The model under review builds one solid part; all positions refer to its coordinate system, in mm. A direction names the side the tool comes from. Give positions to 0.01 mm unless a question says otherwise; leave off trailing zeros. Write each loop counter-clockwise with the first axis right and the second up, starting at its lowest first coordinate (ties: lowest second). Pieces come first, ordered by that corner, then holes. Notation, with made-up numbers: (-21.5, 70.5) -> (-7.5, 70.5) arc R13 cw to (-7.5, 80.5) -> close; hole circle Ø11 at (-7.75, 54.25). An arc over 180 degrees is marked (long way). Use CSV: the item, a comma, the result in double quotes.
Autodesk Inventor part; units mm, degrees
ref_plane "YZ Plane" through (0, 0, 0) normal (1, 0, 0) x (0, 1, 0)
ref_plane "XZ Plane" through (0, 0, 0) normal (0, 1, 0) x (-1, 0, 0)
ref_plane "XY Plane" through (0, 0, 0) normal (0, 0, 1) x (1, 0, 0)
ref_plane "Work Plane1" through (0, 0, 0) normal (0, 0, 1) x (1, 0, 0)
sketch "Sketch1" plane through (0, 0, 0) normal (0, 0, 1) x (1, 0, 0)
  arc A0 (-10.7354, 13.2764) -> (-8.7899, 5.3181) centre (6.5146, 13.2764) ccw
  line L0 (2.2646, -15.9406) -> (-8.7899, 5.3181)
  line L1 (2.2646, -15.9406) -> (17.0046, -15.9406)
  line L2 (17.0046, -15.9406) -> (17.0046, -1.0343)
  arc A1 (-5.2391, 19.424) -> (17.0046, -1.0343) centre (26.9358, 32.085) ccw
  arc A2 (-5.2391, 19.424) -> (-10.7354, 23.5341) centre (-10.7011, 17.8498) ccw
  line L3 (-10.7354, 23.5341) -> (-10.7354, 13.2764)
  line L4 (17.0046, -15.9406) -> (26.0046, -15.9406)
  line L5 (26.0046, -15.9406) -> (26.0046, 2.0594)
  line L6 (26.0046, 2.0594) -> (17.0046, 2.0594)
  line L7 (17.0046, 2.0594) -> (17.0046, -15.9406)
  line L8 (17.0046, -15.9406) -> (8.0046, -15.9406)
  line L9 (8.0046, -15.9406) -> (8.0046, 2.0594)
  line L10 (8.0046, 2.0594) -> (17.0046, 2.0594)
  line L11 (17.0046, 2.0594) -> (17.0046, -15.9406)
  point P0 (0, 0)
  dimension "d0" = 9
  dimension "d1" = 18
  dimension "d2" = 9
extrude "Extrusion1" add sketch "Sketch1" along normal blind 6 contours L9 L10 A1 L2 L1 | L10 L7 A1 | L2 L7 L6 L5 L4
sketch "Sketch2" plane through (0, 0, 6) normal (0, 0, 1) x (1, 0, 0)
  line L0 (26.0046, 2.0594) -> (8.0046, 2.0594)
  line L1 (8.0046, 2.0594) -> (8.0046, -15.9406)
  line L2 (8.0046, -15.9406) -> (26.0046, -15.9406)
  line L3 (26.0046, -15.9406) -> (26.0046, 2.0594)
  line L4 (17.0046, -15.9406) -> (17.0046, -12.4406) construction
  line L5 (17.0046, -12.4406) -> (17.0046, -2.4406) construction
  point P0 (0, 0)
  dimension "d5" = 3.5
  dimension "d6" = 10
hole "Hole1" at (17.0046, -12.4406, 6) at (17.0046, -2.4406, 6) direction (0, 0, -1) diameter 3 end through all
sketch "Sketch3" plane through (0, 0, 0) normal (0, 0, -1) x (-1, 0, 0)
  circle A0 centre (-17.0046, -12.4406) radius 1.5
  circle A1 centre (-17.0046, -2.4406) radius 1.5
  line L0 (-8.0046, -15.9406) -> (-26.0046, -15.9406)
  line L1 (-8.0046, 2.0594) -> (-8.0046, -15.9406)
  line L2 (-26.0046, 2.0594) -> (-8.0046, 2.0594)
  line L3 (-26.0046, -15.9406) -> (-26.0046, 2.0594)
  line L4 (-20.2955, -12.4406) -> (-18.65, -9.5906)
  line L5 (-18.65, -9.5906) -> (-15.3591, -9.5906)
  line L6 (-15.3591, -9.5906) -> (-13.7137, -12.4406)
  line L7 (-13.7137, -12.4406) -> (-15.3591, -15.2906)
  line L8 (-15.3591, -15.2906) -> (-18.65, -15.2906)
  line L9 (-18.65, -15.2906) -> (-20.2955, -12.4406)
  line L10 (-20.2955, -2.4406) -> (-18.65, 0.4094)
  line L11 (-18.65, 0.4094) -> (-15.3591, 0.4094)
  line L12 (-15.3591, 0.4094) -> (-13.7137, -2.4406)
  line L13 (-13.7137, -2.4406) -> (-15.3591, -5.2906)
  line L14 (-15.3591, -5.2906) -> (-18.65, -5.2906)
  line L15 (-18.65, -5.2906) -> (-20.2955, -2.4406)
  point P0 (0, 0)
  dimension "d14" = 5.7
ref_plane "Work Plane2" through (0, 0, 3.5) normal (0, 0, -1) x (-1, 0, 0)
sketch "Sketch4" plane through (0, 0, 3.5) normal (0, 0, -1) x (-1, 0, 0)
  line L0 (-18.65, 0.4094) -> (-15.3591, 0.4094)
  line L1 (-20.2955, -2.4406) -> (-18.65, 0.4094)
  circle A0 centre (-17.0046, -2.4406) radius 1.5
  circle A1 centre (-17.0046, -12.4406) radius 1.5
  line L2 (-15.3591, -5.2906) -> (-18.65, -5.2906)
  line L3 (-18.65, -9.5906) -> (-15.3591, -9.5906)
  line L4 (-20.2955, -12.4406) -> (-18.65, -9.5906)
  line L5 (-20.2955, -12.4406) -> (-18.65, -9.5906)
  line L6 (-18.65, -9.5906) -> (-15.3591, -9.5906)
  line L7 (-15.3591, -9.5906) -> (-13.7137, -12.4406)
  line L8 (-13.7137, -12.4406) -> (-15.3591, -15.2906)
  line L9 (-15.3591, -15.2906) -> (-18.65, -15.2906)
  line L10 (-18.65, -15.2906) -> (-20.2955, -12.4406)
  line L11 (-20.2955, -2.4406) -> (-18.65, 0.4094)
  line L12 (-18.65, 0.4094) -> (-15.3591, 0.4094)
  line L13 (-15.3591, 0.4094) -> (-13.7137, -2.4406)
  line L14 (-13.7137, -2.4406) -> (-15.3591, -5.2906)
  line L15 (-15.3591, -5.2906) -> (-18.65, -5.2906)
  line L16 (-18.65, -5.2906) -> (-20.2955, -2.4406)
  point P0 (0, 0)
extrude "Extrusion2" cut sketch "Sketch3" against normal blind 4 contours L4 L5 L6 L7 L8 L9 | L10 L11 L12 L13 L14 L15
properties part number "holder"
Q1. To check wall thickness, follow probe 1 along Y at (x, z) = (17.5, 0.85); probe 2 along Y at (x, z) = (19.5, 1.55); probe 3 along X at (y, z) = (-14.75, 2). State the ranges of each line that lie inside material, in increasing order.
Derived:
probe 1,"y = -15.94 to -15.29, -9.59 to -5.29, 0.41 to 2.06"
probe 2,"y = -15.94 to -13.82, -11.06 to -3.82, -1.06 to 2.06"
probe 3,"x = 8 to 15.05, 18.96 to 26"
Q2. The part is to be moulded in two halves that separate along X. For faces 3 (the flat face through (14.548, -10.996, 1.972)), 4 (the flat face through (17, -7, 6)), 5 (the flat face through (26.005, -7, 3)), say which applies: pulls with the +X half, pulls with the -X half, needs draft (parallel to the pull), parting line crosses it, or undercut.
Derived:
face 3,"undercut"
face 4,"needs draft"
face 5,"pulls with the +X half"
Q3. Consider section C-C (x = 18.25). Write out the cut boundary in (y, z).
Derived:
outline,"(-15.94, 0) -> (-15.29, 0) -> (-15.29, 4) -> (-13.28, 4) -> (-13.28, 6) -> (-15.94, 6) -> close; (-11.6, 4) -> (-9.59, 4) -> (-9.59, 0) -> (-5.29, 0) -> (-5.29, 4) -> (-3.28, 4) -> (-3.28, 6) -> (-11.6, 6) -> close; (-1.6, 4) -> (0.41, 4) -> (0.41, 0) -> (2.06, 0) -> (2.06, 6) -> (-1.6, 6) -> close"
Q4. Machinability: for faces 1 (the flat face through (19.46, -3.89, 1.97)), 2 (the flat face through (17, -7, 0)), which of the approach directions +Z, -Z, +X, -X, +Y, -Y give a long, thin tool a straight path to every point of the face, cutting with its end or side? Answer none if there is none.
Derived:
face 1,"-Z"
face 2,"-Z, +X, -X, +Y, -Y"
Q5. Consider section B-B (y = -13). Write out the cut boundary in (x, z), then the cut area to 3 significant figures.
Derived:
outline,"(8, 0) -> (14.04, 0) -> (14.04, 4) -> (15.61, 4) -> (15.61, 6) -> (8, 6) -> close; (18.4, 4) -> (19.97, 4) -> (19.97, 0) -> (26, 0) -> (26, 6) -> (18.4, 6) -> close"
area,"78.7 mm2"
Q6. Consider section A-A (z = 1). Write out the cut boundary in (x, y).
Derived:
outline,"(8, -15.94) -> (26, -15.94) -> (26, 2.06) -> (8, 2.06) -> close; hole (13.71, -12.44) -> (15.36, -15.29) -> (18.65, -15.29) -> (20.3, -12.44) -> (18.65, -9.59) -> (15.36, -9.59) -> close; hole (13.71, -2.44) -> (15.36, -5.29) -> (18.65, -5.29) -> (20.3, -2.44) -> (18.65, 0.41) -> (15.36, 0.41) -> close"
Q7. Insertion check: pin 1 (5 mm diameter, centred on x = 17, y = -12.44, fed in from -Z); pin 2 (2.5 mm diameter, centred on x = 17, y = -2.44, fed in from +Z). Each pin has a flat end and moves straight along its axis. Give the tip position at first contact, or say it passes through.
Derived:
pin 1,"stops at z = 4"
pin 2,"passes through"
Q8. Consider section D-D (x = 14.5). Write out the cut boundary in (y, z).
Derived:
outline,"(-15.94, 0) -> (-13.8, 0) -> (-13.8, 4) -> (-11.08, 4) -> (-11.08, 0) -> (-3.8, 0) -> (-3.8, 4) -> (-1.08, 4) -> (-1.08, 0) -> (2.06, 0) -> (2.06, 6) -> (-15.94, 6) -> close"
